For this review, take the finished solid that the model builds, in its own axes (mm). Round coordinates to 2 decimals unless told otherwise and drop trailing zeros. Write each loop counter-clockwise with the first axis right and the second up, starting at its lowest first coordinate (ties: lowest second). Pieces come first, ordered by that corner, then holes. Notation, with made-up numbers: M 11,-3 L 24,-3 A12 cw 24,8 Z; hole C 48.5,-24 d2. An arc over 180 degrees is marked long. Answer in a Markdown table with one row per item.
```python
from build123d import *
from OCP.BRepFilletAPI import BRepFilletAPI_MakeChamfer

# Parameters (mm, degrees)
SKETCH_1_W           = 276
SKETCH_1_H           = 276
EXTRUDE_1_DEPTH      = 6
SKETCH_4_R           = 6.5
SKETCH_4_R_2         = 2
CUT_EXTRUDE_1_DEPTH  = 10
SKETCH_5_R           = 2.4
CUT_EXTRUDE_2_DEPTH  = 196.253681143
FILLET_1_R           = 110
EXTRUDE_1_2_DEPTH    = 5
CHAMFER_2_SIZE       = 1.5
CHAMFER_2_SIZE2      = 4.121216129
SKETCH_9_W           = 33
SKETCH_9_H           = 33
EXTRUDE_2_DEPTH      = 11
FILLET_2_R           = 1
FILLET_3_R           = 10
CHAMFER_5_SIZE       = 3
CHAMFER_5_SIZE2      = 5.196152423
SKETCH_6_R           = 103
CUT_EXTRUDE_3_DEPTH  = 10
CHAMFER_6_SIZE       = 2
SKETCH_13_R          = 4.5
CUT_EXTRUDE_6_DEPTH  = 196.47122551
SKETCH_14_R          = 6
CUT_EXTRUDE_7_DEPTH  = 5
SKETCH_15_R          = 7
CUT_EXTRUDE_8_DEPTH  = 3
SKETCH_16_R          = 8.5
CUT_EXTRUDE_9_DEPTH  = 2
CHAMFER_7_SIZE       = 0.5
SKETCH_18_W          = 167.450202049
SKETCH_18_H          = 12.846548741
SKETCH_18_W_2        = 47.896370642
SKETCH_18_H_2        = 198.133814491
CUT_EXTRUDE_10_DEPTH = 196.900484949


# Read off the part's stored shape, not the designer's step: Вытянуть-Тонкостенный1
with BuildPart() as part:
    # Эскиз1 → Extrude 1 (new body)
    with BuildSketch(Plane(origin=(0, 0, 0), x_dir=(1, 0, 0), z_dir=(0, 1, 0))):
        Rectangle(SKETCH_1_W, SKETCH_1_H)
    extrude(amount=EXTRUDE_1_DEPTH)

    # Эскиз4 → Cut-Extrude 1 (cut)
    with BuildSketch(Plane(origin=(0, 6, 0), x_dir=(1, 0, 0), z_dir=(0, 1, 0))):
        with Locations(Location((66, 114, 0), (0, 0, 270))):
            Circle(SKETCH_4_R)
        with Locations(Location((-120, 0, 0), (0, 0, 270))):
            Circle(SKETCH_4_R_2)
        with Locations(Location((66, -114, 0), (0, 0, 90))):
            Circle(SKETCH_4_R)
    extrude(amount=-CUT_EXTRUDE_1_DEPTH, mode=Mode.SUBTRACT)

    # Эскиз5 → Вырез-Вытянуть2 (cut, through all)
    with BuildSketch(Plane(origin=(0, 6, 0), x_dir=(1, 0, 0), z_dir=(0, 1, 0))):
        with Locations(Location((-85, 85, 0), (0, 0, 270))):
            Circle(SKETCH_5_R)
        with Locations(Location((85, 85, 0), (0, 0, 270))):
            Circle(SKETCH_5_R)
        with Locations(Location((85, -85, 0), (0, 0, 270))):
            Circle(SKETCH_5_R)
        with Locations(Location((-85, -85, 0), (0, 0, 270))):
            Circle(SKETCH_5_R)
        with Locations(Location((-90, 0, 0), (0, 0, 270))):
            Circle(SKETCH_5_R)
        with Locations(Location((0, 90, 0), (0, 0, 270))):
            Circle(SKETCH_5_R)
        with Locations(Location((0, -90, 0), (0, 0, 90))):
            Circle(SKETCH_5_R)
        with Locations(Location((90, 0, 0), (0, 0, 90))):
            Circle(SKETCH_5_R)
    extrude(amount=-CUT_EXTRUDE_2_DEPTH, mode=Mode.SUBTRACT)

    # Скругление1
    fillet_1_edges = [part.edges().sort_by_distance(p)[0] for p in [
        (138, 3, 138),
        (-138, 3, 138),
        (-138, 3, -138),
        (138, 3, -138),
    ]]
    fillet(fillet_1_edges, radius=FILLET_1_R)

    # Extrude 1 2 outline → Extrude 1 2 (add)
    # profile 1 of 2: a face of its own
    with BuildSketch(Plane(origin=(0, 6, 0), x_dir=(1, 0, 0), z_dir=(0, 1, 0))):
        Polygon((80.1, -105.859361204), (66, -97.718722409), (51.9, -105.859361204), (51.9, -122.140638796), (66, -130.281277591), (80.1, -122.140638796), align=None)
        Polygon((56.9, -108.74611255), (66, -103.492225101), (75.1, -108.74611255), (75.1, -119.25388745), (66, -124.507774899), (56.9, -119.25388745), align=None, mode=Mode.SUBTRACT)
    # profile 2 of 2: a face of its own
    with BuildSketch(Plane(origin=(0, 6, 0), x_dir=(1, 0, 0), z_dir=(0, 1, 0))):
        Polygon((51.9, 122.140638796), (51.9, 105.859361204), (66, 97.718722409), (80.1, 105.859361204), (80.1, 122.140638796), (66, 130.281277591), align=None)
        Polygon((66, 103.492225101), (56.9, 108.74611255), (56.9, 119.25388745), (66, 124.507774899), (75.1, 119.25388745), (75.1, 108.74611255), align=None, mode=Mode.SUBTRACT)
    extrude(amount=EXTRUDE_1_2_DEPTH)

    # Фаска2: one chamfer whose edges measure the first distance from different faces: ONE call of the kernel's chamfer builder (chamfer() names one face for all edges)
    chamfer_2_edges_1 = [part.edges().sort_by_distance(p)[0] for p in [
        (70.55, 11, 106.119168825),
        (61.45, 11, 106.119168825),
        (56.9, 11, 114),
        (61.45, 11, 121.880831175),
        (70.55, 11, 121.880831175),
        (75.1, 11, 114),
    ]]
    chamfer_2_side_1 = [part.faces().sort_by_distance(p)[0] for p in [
        (72.834618942, 11, 102.162092741),
    ]]
    chamfer_2_edges_2 = [part.edges().sort_by_distance(p)[0] for p in [
        (75.1, 11, -114),
        (70.55, 11, -121.880831175),
        (61.45, 11, -121.880831175),
        (56.9, 11, -114),
        (61.45, 11, -106.119168825),
        (70.55, 11, -106.119168825),
    ]]
    chamfer_2_side_2 = [part.faces().sort_by_distance(p)[0] for p in [
        (52.330762115, 11, -114),
    ]]
    chamfer_2 = BRepFilletAPI_MakeChamfer(part.part.solid().wrapped)
    for e in chamfer_2_edges_1:
        chamfer_2.Add(CHAMFER_2_SIZE, CHAMFER_2_SIZE2, e.wrapped, chamfer_2_side_1[0].wrapped)  # the first distance lies on this face
    for e in chamfer_2_edges_2:
        chamfer_2.Add(CHAMFER_2_SIZE, CHAMFER_2_SIZE2, e.wrapped, chamfer_2_side_2[0].wrapped)  # the first distance lies on this face
    add(Compound.cast(chamfer_2.Shape()), mode=Mode.REPLACE)

    # Эскиз9 → Бобышка-Вытянуть2 (add)
    with BuildSketch(Plane(origin=(0, 6, 0), x_dir=(1, 0, 0), z_dir=(0, 1, 0))):
        with Locations((-120, 0)):
            Rectangle(SKETCH_9_W, SKETCH_9_H)
    extrude(amount=EXTRUDE_2_DEPTH)

    # Эскиз10 → Вырез-Повернуть1 (revolve, cut)
    with BuildSketch(Plane(origin=(0, 13, 0), x_dir=(1, 0, 0), z_dir=(0, 1, 0))):
        with BuildLine():
            Line((-131.6, 0), (-108.4, 0))
            ThreePointArc((-108.4, 0), (-120, 11.6), (-131.6, 0))
        make_face()
    revolve(axis=Axis((-131.6, 13, 0), (1, 0, 0)), mode=Mode.SUBTRACT)

    # Скругление2
    fillet_2_edges = [part.edges().sort_by_distance(p)[0] for p in [
        (-119.999999999, 1.573714514, -1.999999986),
        (-120, 17, -10.888526071),
    ]]
    fillet(fillet_2_edges, radius=FILLET_2_R)

    # Скругление3
    fillet_3_edges = [part.edges().sort_by_distance(p)[0] for p in [
        (-103.5, 11.5, 16.5),
        (-103.5, 11.5, -16.5),
        (-136.5, 11.5, -16.5),
        (-136.5, 11.5, 16.5),
    ]]
    fillet(fillet_3_edges, radius=FILLET_3_R)

    # Фаска5
    chamfer_5_edges = [part.edges().sort_by_distance(p)[0] for p in [
        (66, 0, 120.5),
        (66, 0, -120.5),
    ]]
    chamfer_5_side = [part.faces().sort_by_distance(p)[0] for p in [
        (-0.244968045, 0, 0),
    ]]
    chamfer(chamfer_5_edges, length=CHAMFER_5_SIZE, length2=CHAMFER_5_SIZE2, reference=chamfer_5_side[0])

    # Эскиз6 → Вырез-Вытянуть3 (cut)
    with BuildSketch(Plane(origin=(0, 6, 0), x_dir=(1, 0, 0), z_dir=(0, 1, 0))):
        with Locations(Location((0, 0, 0), (0, 0, 270))):
            Circle(SKETCH_6_R)
    extrude(amount=-CUT_EXTRUDE_3_DEPTH, mode=Mode.SUBTRACT)

    # Фаска6
    chamfer_6_edges = [part.edges().sort_by_distance(p)[0] for p in [
        (85, 6, -87.4),
        (85, 6, 82.6),
        (-85, 6, 82.6),
        (-85, 6, -87.4),
    ]]
    chamfer(chamfer_6_edges, length=CHAMFER_6_SIZE)

    # Эскиз13 → Вырез-Вытянуть6 (cut, through all)
    with BuildSketch(Plane(origin=(0, 6, 0), x_dir=(1, 0, 0), z_dir=(0, 1, 0))):
        with Locations(Location((112, 50, 0), (0, 0, 270))):
            Circle(SKETCH_13_R)
        with Locations(Location((112, -50, 0), (0, 0, 90))):
            Circle(SKETCH_13_R)
    extrude(amount=-CUT_EXTRUDE_6_DEPTH, mode=Mode.SUBTRACT)

    # Эскиз14 → Вырез-Вытянуть7 (cut)
    with BuildSketch(Plane(origin=(0, 6, 0), x_dir=(1, 0, 0), z_dir=(0, 1, 0))):
        with Locations(Location((112, 50, 0), (0, 0, 270))):
            Circle(SKETCH_14_R)
        with Locations(Location((112, -50, 0), (0, 0, 90))):
            Circle(SKETCH_14_R)
    extrude(amount=-CUT_EXTRUDE_7_DEPTH, mode=Mode.SUBTRACT)

    # Эскиз15 → Вырез-Вытянуть8 (cut)
    with BuildSketch(Plane(origin=(0, 6, 0), x_dir=(1, 0, 0), z_dir=(0, 1, 0))):
        with Locations(Location((112, 50, 0), (0, 0, 270))):
            Circle(SKETCH_15_R)
        with Locations(Location((112, -50, 0), (0, 0, 90))):
            Circle(SKETCH_15_R)
    extrude(amount=-CUT_EXTRUDE_8_DEPTH, mode=Mode.SUBTRACT)

    # Эскиз16 → Вырез-Вытянуть9 (cut)
    with BuildSketch(Plane(origin=(0, 6, 0), x_dir=(1, 0, 0), z_dir=(0, 1, 0))):
        with Locations(Location((112, 50, 0), (0, 0, 270))):
            Circle(SKETCH_16_R)
        with Locations(Location((112, -50, 0), (0, 0, 90))):
            Circle(SKETCH_16_R)
    extrude(amount=-CUT_EXTRUDE_9_DEPTH, mode=Mode.SUBTRACT)

    # Фаска7
    chamfer_7_edges = [part.edges().sort_by_distance(p)[0] for p in [
        (112, 1, -54.5),
        (112, 1, 54.5),
        (112, 3, -56),
        (112, 3, 56),
        (112, 6, -58.5),
        (112, 4, -57),
        (112, 4, 57),
        (112, 6, 58.5),
    ]]
    chamfer(chamfer_7_edges, length=CHAMFER_7_SIZE)

    # Эскиз18 → Вырез-Вытянуть10 (cut, through all)
    with BuildSketch(Plane(origin=(0, 17, 0), x_dir=(1, 0, 0), z_dir=(0, 1, 0))):
        with Locations((-6.548331924, 137.42327437)):
            Rectangle(SKETCH_18_W, SKETCH_18_H)
        with Locations((-6.548331924, -137.42327437)):
            Rectangle(SKETCH_18_W, SKETCH_18_H)
        with Locations((154.948185321, -9.822497885)):
            Rectangle(SKETCH_18_W_2, SKETCH_18_H_2)
    extrude(amount=-CUT_EXTRUDE_10_DEPTH, mode=Mode.SUBTRACT)


solid = part.part
```
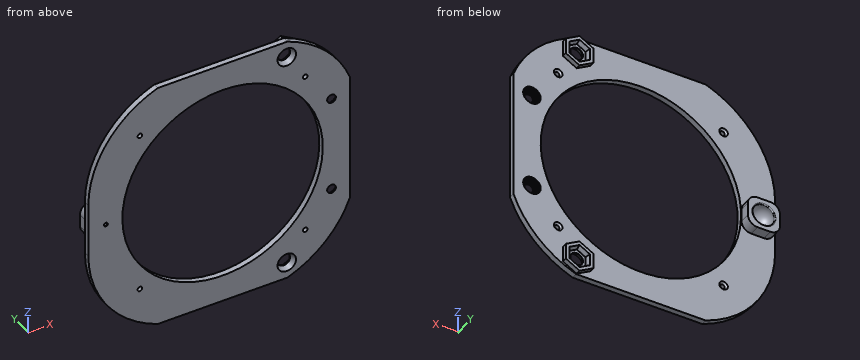
Q1. Take a section at C-C (z = 50). State how many separate pieces and enclosed holes the cut face has, then the cut area to 3 significant figures.
Found:
| item | result |
|---|---|
| separate pieces | 3 |
| enclosed holes | 0 |
| area | 438 mm² |
Q2. Take a section at D-D (x = 36). State the section outline as (y, z) points, then the cut area to 3 significant figures.
Found:
| item | result |
|---|---|
| outline | M 0,-131 L 6,-131 L 6,-96.5 L 0,-96.5 Z; M 0,96.5 L 6,96.5 L 6,131 L 0,131 Z |
| area | 414 mm² |
Q3. For probe 1 along X at (y, z) = (0.5, 0); probe 2 along X at (y, z) = (2.4, -85); probe 3 along X at (y, z) = (3.4, 50), list the stretches that pass through material, from the lowest coordinate up.
Found:
| item | result |
|---|---|
| probe 1 | -138 to -122, -118 to -103, 103 to 131 |
| probe 2 | -122.08 to -87.4, -82.6 to -58.17, 58.17 to 82.6, 87.4 to 122.08 |
| probe 3 | -135.78 to -90.05, 90.05 to 105, 119 to 131 |
Q4. Take a section at A-A (z = -114). State the section outline as (x, y) points.
Found:
| item | result |
|---|---|
| outline | M -96.59,0 L 56.5,0 L 59.5,5.2 L 59.5,6 L 56.9,6 L 56.9,6.88 L 55.4,11 L 51.9,11 L 51.9,6 L -96.59,6 Z; M 72.5,5.2 L 75.5,0 L 96.59,0 L 96.59,6 L 80.1,6 L 80.1,11 L 76.6,11 L 75.1,6.88 L 75.1,6 L 72.5,6 Z |
Q5. Insertion check: P1, Ø1, axis at y = 5, z = -40, coming from the -X side; P2, Ø0.7, axis at y = 6.5, z = -113.5, coming from the +X side; P3, Ø3.5, axis at x = 112.5, z = 52, coming from the +Y side; P4, Ø13.5, axis at x = 110, z = -46, coming from the +Y side. Each pin has a flat end and moves straight along its axis. Give the tip position at first contact, or say it passes through.
Found:
| item | result |
|---|---|
| P1 | x = -137.4 |
| P2 | x = 80.1 |
| P3 | through |
| P4 | y = 6 |
Q6. Take a section at B-B (x = -3.5). State the section outline as (y, z) points, then the cut area to 3 significant figures.
Found:
| item | result |
|---|---|
| outline | M 0,-131 L 6,-131 L 6,-102.94 L 0,-102.94 Z; M 0,102.94 L 6,102.94 L 6,131 L 0,131 Z |
| area | 337 mm² |
